```python
from build123d import *
from build123d.topology import SkipClean

# Parameters (mm, degrees)
SKETCH1_W                      = 390
SKETCH1_H                      = 3
BOSS_EXTRUDE1_DEPTH            = 5
DRAFT1_ANGLE                   = -15
CIRPATTERN1_COUNT              = 12
DRAFT1_OF_CIRPATTERN1_2_ANGLE  = -15
DRAFT1_OF_CIRPATTERN1_3_ANGLE  = -15
DRAFT1_OF_CIRPATTERN1_4_ANGLE  = -15
DRAFT1_OF_CIRPATTERN1_5_ANGLE  = -15
DRAFT1_OF_CIRPATTERN1_6_ANGLE  = -15
DRAFT1_OF_CIRPATTERN1_7_ANGLE  = -15
DRAFT1_OF_CIRPATTERN1_8_ANGLE  = -15
DRAFT1_OF_CIRPATTERN1_9_ANGLE  = -15
DRAFT1_OF_CIRPATTERN1_10_ANGLE = -15
DRAFT1_OF_CIRPATTERN1_11_ANGLE = -15
DRAFT1_OF_CIRPATTERN1_12_ANGLE = -15
SKETCH3_OUTSIDE_W              = 265.338
SKETCH3_OUTSIDE_H              = 265.338
CUT_EXTRUDE1_DEPTH             = 563.983125857


# Read off the part's stored shape, not the designer's step: CSK for M4 Countersunk Flat Head Screw1
with BuildPart() as part:
    # Sketch1 → Revolve1 (revolve)
    with BuildSketch(Plane.XY, mode=Mode.PRIVATE) as revolve1_sk:
        with Locations((355, 83.5)):
            Rectangle(SKETCH1_W, SKETCH1_H)
    revolve(revolve1_sk.sketch.rotate(Axis((0, 0, 0), (1, 0, 0)), 90), axis=Axis((0, 0, 0), (1, 0, 0)))

    # Sketch2 → Boss-Extrude1 (add, symmetric)
    with BuildSketch(Plane(origin=(155, 0, 0), x_dir=(0, 0, -1), z_dir=(1, 0, 0))):
        with BuildLine():
            Line((10.703147762, 81.298478633), (11.094726339, 84.272813217))
            ThreePointArc((11.094726339, 84.272813217), (0, 85), (-11.094726339, 84.272813217))
            Line((-11.094726339, 84.272813217), (-10.703147762, 81.298478633))
            ThreePointArc((-10.703147762, 81.298478633), (0, 82), (10.703147762, 81.298478633))
        make_face()
    boss_extrude1 = extrude(amount=BOSS_EXTRUDE1_DEPTH, both=True)

    # Draft1
    draft1_faces = [part.faces().sort_by_distance(p)[0] for p in [
        (155, 82.785645925, 10.89893705),
        (155, 82.785645925, -10.89893705),
    ]]
    draft(draft1_faces, Plane(origin=(155, 0, 0), x_dir=(0, 0, 1), z_dir=(1, 0, 0)), DRAFT1_ANGLE)

    # CirPattern1: Boss-Extrude1 ×12 about axis
    with SkipClean():  # the faces are left unmerged after this step: merging them gives an invalid solid
        cirpattern1_axis = Axis((0, 0, 0), (1, 0, 0))
        for i in range(1, CIRPATTERN1_COUNT):
            add(boss_extrude1.rotate(cirpattern1_axis, i * 360 / CIRPATTERN1_COUNT))

    # Draft1 of CirPattern1 2
    draft1_of_cirpattern1_2_faces = [part.faces().sort_by_distance(p)[0] for p in [
        (155, 66.245003914, 50.831579322),
        (155, 77.143940965, 31.954066602),
    ]]
    draft(draft1_of_cirpattern1_2_faces, Plane(origin=(155, 0, 0), x_dir=(0, -0.49999999999999994, 0.8660254037844387), z_dir=(1, 0, 0)), DRAFT1_OF_CIRPATTERN1_2_ANGLE)

    # Draft1 of CirPattern1 3
    draft1_of_cirpattern1_3_faces = [part.faces().sort_by_distance(p)[0] for p in [
        (155, 31.954066602, 77.143940965),
        (155, 50.831579322, 66.245003914),
    ]]
    draft(draft1_of_cirpattern1_3_faces, Plane(origin=(155, 0, 0), x_dir=(0, -0.8660254037844386, 0.5000000000000001), z_dir=(1, 0, 0)), DRAFT1_OF_CIRPATTERN1_3_ANGLE)

    # Draft1 of CirPattern1 4
    draft1_of_cirpattern1_4_faces = [part.faces().sort_by_distance(p)[0] for p in [
        (155, -10.89893705, 82.785645925),
        (155, 10.89893705, 82.785645925),
    ]]
    draft(draft1_of_cirpattern1_4_faces, Plane(origin=(155, 0, 0), x_dir=(0, -1, 0), z_dir=(1, 0, 0)), DRAFT1_OF_CIRPATTERN1_4_ANGLE)

    # Draft1 of CirPattern1 5
    draft1_of_cirpattern1_5_faces = [part.faces().sort_by_distance(p)[0] for p in [
        (155, -50.831579322, 66.245003914),
        (155, -31.954066602, 77.143940965),
    ]]
    draft(draft1_of_cirpattern1_5_faces, Plane(origin=(155, 0, 0), x_dir=(0, -0.8660254037844387, -0.4999999999999998), z_dir=(1, 0, 0)), DRAFT1_OF_CIRPATTERN1_5_ANGLE)

    # Draft1 of CirPattern1 6
    draft1_of_cirpattern1_6_faces = [part.faces().sort_by_distance(p)[0] for p in [
        (155, -77.143940965, 31.954066602),
        (155, -66.245003914, 50.831579322),
    ]]
    draft(draft1_of_cirpattern1_6_faces, Plane(origin=(155, 0, 0), x_dir=(0, -0.49999999999999994, -0.8660254037844387), z_dir=(1, 0, 0)), DRAFT1_OF_CIRPATTERN1_6_ANGLE)

    # Draft1 of CirPattern1 7
    draft1_of_cirpattern1_7_faces = [part.faces().sort_by_distance(p)[0] for p in [
        (155, -82.785645925, -10.89893705),
        (155, -82.785645925, 10.89893705),
    ]]
    draft(draft1_of_cirpattern1_7_faces, Plane(origin=(155, 0, 0), x_dir=(0, 0, -1), z_dir=(1, 0, 0)), DRAFT1_OF_CIRPATTERN1_7_ANGLE)

    # Draft1 of CirPattern1 8
    draft1_of_cirpattern1_8_faces = [part.faces().sort_by_distance(p)[0] for p in [
        (155, -66.245003914, -50.831579322),
        (155, -77.143940965, -31.954066602),
    ]]
    draft(draft1_of_cirpattern1_8_faces, Plane(origin=(155, 0, 0), x_dir=(0, 0.5000000000000001, -0.8660254037844386), z_dir=(1, 0, 0)), DRAFT1_OF_CIRPATTERN1_8_ANGLE)

    # Draft1 of CirPattern1 9
    draft1_of_cirpattern1_9_faces = [part.faces().sort_by_distance(p)[0] for p in [
        (155, -31.954066602, -77.143940965),
        (155, -50.831579322, -66.245003914),
    ]]
    draft(draft1_of_cirpattern1_9_faces, Plane(origin=(155, 0, 0), x_dir=(0, 0.8660254037844384, -0.5000000000000004), z_dir=(1, 0, 0)), DRAFT1_OF_CIRPATTERN1_9_ANGLE)

    # Draft1 of CirPattern1 10
    draft1_of_cirpattern1_10_faces = [part.faces().sort_by_distance(p)[0] for p in [
        (155, 10.89893705, -82.785645925),
        (155, -10.89893705, -82.785645925),
    ]]
    draft(draft1_of_cirpattern1_10_faces, Plane.YZ.offset(155), DRAFT1_OF_CIRPATTERN1_10_ANGLE)

    # Draft1 of CirPattern1 11
    draft1_of_cirpattern1_11_faces = [part.faces().sort_by_distance(p)[0] for p in [
        (155, 50.831579322, -66.245003914),
        (155, 31.954066602, -77.143940965),
    ]]
    draft(draft1_of_cirpattern1_11_faces, Plane(origin=(155, 0, 0), x_dir=(0, 0.8660254037844386, 0.5000000000000001), z_dir=(1, 0, 0)), DRAFT1_OF_CIRPATTERN1_11_ANGLE)

    # Draft1 of CirPattern1 12
    draft1_of_cirpattern1_12_faces = [part.faces().sort_by_distance(p)[0] for p in [
        (155, 77.143940965, -31.954066602),
        (155, 66.245003914, -50.831579322),
    ]]
    draft(draft1_of_cirpattern1_12_faces, Plane(origin=(155, 0, 0), x_dir=(0, 0.5000000000000004, 0.8660254037844384), z_dir=(1, 0, 0)), DRAFT1_OF_CIRPATTERN1_12_ANGLE)

    # Sketch3 outside → Cut-Extrude1 (cut, through all)
    with SkipClean():  # the faces are left unmerged after this step: merging them gives an invalid solid
        with BuildSketch(Plane(origin=(0, 0, 0), x_dir=(0, 0, -1), z_dir=(1, 0, 0))):
            Rectangle(SKETCH3_OUTSIDE_W, SKETCH3_OUTSIDE_H)
            with BuildLine():
                Line((0, 0), (-85, 0))
                ThreePointArc((-85, 0), (0, 85), (85, 0))
                Line((85, 0), (0, 0))
            make_face(mode=Mode.SUBTRACT)
        extrude(amount=CUT_EXTRUDE1_DEPTH, mode=Mode.SUBTRACT)

    # CSK for M4 Countersunk Flat Head Scr 2 → CSK for M4 Countersunk Flat Head Screw1 (revolve, cut)
    with SkipClean():  # the faces are left unmerged after this step: merging them gives an invalid solid
        with BuildSketch(Plane(origin=(540, 0, 0), x_dir=(1, 0, 0), z_dir=(0, 0, 1))):
            Polygon((4.700033545, 85.000033545), (0, 85.000033545), (0, 81.96910869), (2.25, 81.96910869), (2.25, 82.55), align=None)
        revolve(axis=Axis((540, 0, 0), (0, 1, 0)), mode=Mode.SUBTRACT)

    # CSK for M4 Countersunk Flat Head Scr 3 o → CSK for M4 Countersunk Flat Head Scr 3 (revolve, cut)
    with SkipClean():  # the faces are left unmerged after this step: merging them gives an invalid solid
        with BuildSketch(Plane(origin=(540, 0, 0), x_dir=(1, 0, 0), z_dir=(0, 0.9914448613738104, 0.13052619222005205))):
            Polygon((4.700071897, 85.000071897), (0, 85.000071897), (0, 81.96910869), (2.25, 81.96910869), (2.25, 82.55), align=None)
        revolve(axis=Axis((540, 0, 0), (0, 0.13052619222005205, -0.9914448613738104)), mode=Mode.SUBTRACT)

    # CSK for M4 Countersunk Flat Head Scr 4 o → CSK for M4 Countersunk Flat Head Scr 4 (revolve, cut)
    with SkipClean():  # the faces are left unmerged after this step: merging them gives an invalid solid
        with BuildSketch(Plane(origin=(540, 0, 0), x_dir=(1, 0, 0), z_dir=(0, -0.9914448613738104, 0.13052619222005205))):
            Polygon((4.700070707, 85.000070707), (0, 85.000070707), (0, 81.96910869), (2.25, 81.96910869), (2.25, 82.55), align=None)
        revolve(axis=Axis((540, 0, 0), (0, 0.13052619222005205, 0.9914448613738104)), mode=Mode.SUBTRACT)


solid = part.part
```
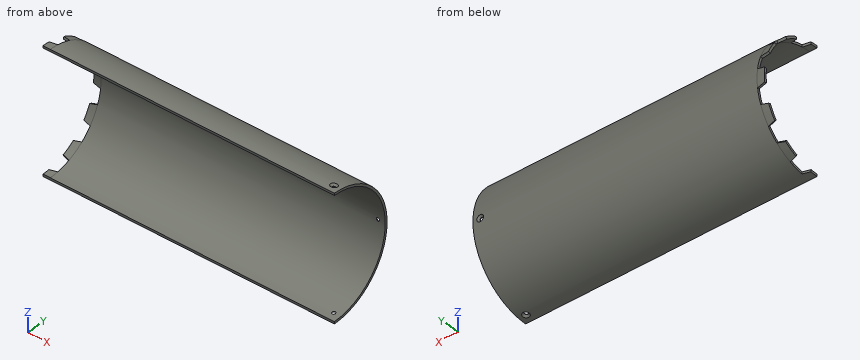
Model file for the job. Use its own axes, mm. Coordinates: 2 decimals unless noted, no trailing zeros. Loops run counter-clockwise (first coordinate to the right, second up) from the corner with the lowest first, then second, coordinate; pieces in that order, holes last. Notation, with made-up numbers: (-9.75, 73.25) - (16.25, 73.25) arc R19 cw to (16.25, 94.25) - close; hole circle Ø2 at (74.5, 26.25). An arc over 180 degrees is marked (long way). Write item = value, one per line. Start each with the question number.
Item 1: Saw through at C-C, the plane x = 195.5. List the corners of the cut face in (y, z).
Item 2: Saw through at A-A, the plane y = 58. List the corners of the cut face in (x, z).
Item 3: Saw through at B-B, the plane y = 20. List the corners of the cut face in (x, z).
Item 4: Wall check: probe 1 along X at (y, z) = (82.15, 0); probe 2 along Z at (x, y) = (377, 12.5); probe 3 along X at (y, z) = (63.5, -55). Give the ranges that are in metal, low to high. Write a range as [from, to].
Item 5: Saw through at D-D, the plane z = 43. List the corners of the cut face in (x, y).
Item 6: Drop flat-ended pins along their axis: pin 1 Ø8 at (x, y) = (496.5, 23) entering from +Z; pin 2 Ø1 at (x, y) = (286.5, 13.5) entering from -Z; pin 3 Ø1 at (x, y) = (240.5, 58.5) entering from -Z. Give the stop position or say it passes through.
Answers:
q1.outline = (0, -85) arc R85 ccw to (0, 85) - (0, 82) arc R82 cw to (0, -82) - close
q2.outline = (160, -62.14) - (550, -62.14) - (550, -57.97) - (160, -57.97) - close; (160, 57.97) - (550, 57.97) - (550, 62.14) - (160, 62.14) - close
q3.outline = (160, -82.61) - (550, -82.61) - (550, -79.52) - (160, -79.52) - close; (160, 79.52) - (550, 79.52) - (550, 82.61) - (160, 82.61) - close
q4.probe_1 = [150, 537.75], [542.25, 550]
q4.probe_2 = [-84.08, -81.04], [81.04, 84.08]
q4.probe_3 = [160, 550]
q5.outline = (150, 69.82) - (550, 69.82) - (550, 73.32) - (150, 73.32) - close
q6.pin_1 = 82.85
q6.pin_2 = -84
q6.pin_3 = -62.14
